from build123d import *

# Parameters (mm, degrees)
SKETCH_R  = 0.48
SKETCH_W  = 22.3
SKETCH_H  = 12.8
PAD_DEPTH = 4.5


with BuildPart() as part:
    # Sketch → Pad (new body)
    with BuildSketch(Plane.XY):
        with BuildLine():
            Line((-17.15, -12.4), (14.15, -12.4))
            ThreePointArc((14.15, -12.4), (16.27132, -11.52132), (17.15, -9.4))
            Line((17.15, -9.4), (17.15, 10.741965))
            ThreePointArc((17.15, 10.741965), (16.27132, 12.863286), (14.15, 13.741965))
            Line((14.15, 13.741965), (-17.15, 13.741965))
            ThreePointArc((-17.15, 13.741965), (-45.41951, 11.467422), (-72.4, 2.727178))
            ThreePointArc((-72.4, 2.727178), (-72.770186, -2.524876), (-68.15, -1e-06))
            ThreePointArc((-17.15, -12.4), (-41.755087, -2.51931), (-68.15, -1e-06))
        make_face()
        with Locations((-13.65, 0)):
            Circle(SKETCH_R, mode=Mode.SUBTRACT)
        with Locations((13.65, 0)):
            Circle(SKETCH_R, mode=Mode.SUBTRACT)
        Rectangle(SKETCH_W, SKETCH_H, mode=Mode.SUBTRACT)
        with BuildLine():
            Line((-17.44, 6.580017), (-17.44, -6.814013))
            ThreePointArc((-19.71, -8.17), (-18.190253, -8.136095), (-17.44, -6.814013))
            ThreePointArc((-19.71, -8.17), (-34.392185, -1.83077), (-49.944735, 1.893553))
            ThreePointArc((-50.141709, 5.809641), (-51.645768, 3.770991), (-49.944735, 1.893553))
            ThreePointArc((-20.45, 9.58), (-35.411915, 8.608801), (-50.141709, 5.809641))
            ThreePointArc((-17.44, 6.580017), (-18.322218, 8.70487), (-20.45, 9.58))
        make_face(mode=Mode.SUBTRACT)
    extrude(amount=PAD_DEPTH)


solid = part.part
Could you check a few things on this model? Use its own coordinates, in mm. A direction names the side the tool comes from. Round coordinates to 2 decimals unless told otherwise and drop trailing zeros. Order: outer loops, then holes, each group sorted by start corner. A loop starts at its lowest first (then second) coordinate and runs counter-clockwise, first axis right, second up.
(1) If we mould it in two halves opening along Y, with no side actions, what happens to faces 1 (the cylindrical face through (-41.39, -2.61, 2.22)), 2 (the flat face through (17.15, 1, 2)), 3 (the cylindrical face through (-51.647, 3.809, 2.218))? For each: released by +Y, released by -Y, zero draft, split by the parting line, or undercut.
Response values:
face 1: released by -Y
face 2: zero draft
face 3: undercut
(2) Imagine slicing it at C-C (x = -32.5). Write out the boundary of the cut face in (y, z), plus the area to 3 significant figures.
Response values:
outline: (-5.29, 0) - (-2.48, 0) - (-2.48, 4.5) - (-5.29, 4.5) - close; (8.94, 0) - (13.33, 0) - (13.33, 4.5) - (8.94, 4.5) - close
area: 32.4 mm2
(3) Imagine slicing it at B-B (x = -5.5). Write out the boundary of the cut face in (y, z).
Response values:
outline: (-12.4, 0) - (-6.4, 0) - (-6.4, 4.5) - (-12.4, 4.5) - close; (6.4, 0) - (13.74, 0) - (13.74, 4.5) - (6.4, 4.5) - close
(4) Imagine slicing it at A-A (z = 1.3). Write out the boundary of the cut face in (x, y), plus the area to 3 significant figures.
Response values:
outline: (-72.4, 2.73) arc R3 ccw (long way) to (-68.15, 0) arc R92.8 cw to (-17.15, -12.4) - (14.15, -12.4) arc R3 ccw to (17.15, -9.4) - (17.15, 10.74) arc R3 ccw to (14.15, 13.74) - (-17.15, 13.74) arc R122 ccw to start; hole (-50.14, 5.81) arc R2 ccw to (-49.94, 1.89) arc R92.8 cw to (-19.71, -8.17) arc R1.54 ccw to (-17.44, -6.81) - (-17.44, 6.58) arc R3 ccw to (-20.45, 9.58) arc R122 ccw to start; hole circle Ø0.96 at (-13.65, 0); hole (-11.15, -6.4) - (11.15, -6.4) - (11.15, 6.4) - (-11.15, 6.4) - close; hole circle Ø0.96 at (13.65, 0)
area: 1,020 mm2
(5) I'm going to push flat-ended pins straight in: pin 1 (1.3 mm diameter, centred on y = 1, z = 1.5, fed in from -X); pin 2 (1.5 mm diameter, centred on x = -2.5, z = 2.5, fed in from +Y); pin 3 (2 mm diameter, centred on x = -64, z = 1.5, fed in from -Y). Where does each tip first touch, or does it pass through?
Response values:
pin 1: stops at x = -74.13
pin 2: stops at y = 13.74
pin 3: stops at y = 0.1
(6) Which directions (+Z, -Z, +X, -X, +Y, -Y) give clear straight access to the entire face, cutting with the end or side of a thin tool? Please do faces 4 (the flat face through (-1, 13.742, 2)), 5 (the flat face through (-2, -12.4, 2)), 6 (the cylindrical face through (-34.18, -1.9, 2.22)).
Response values:
face 4: +Z, -Z, +X, +Y
face 5: +Z, -Z, +X, -X, -Y
face 6: +Z, -Z
(7) Imagine slicing it at D-D (y = 12). Write out the boundary of the cut face in (x, z).
Response values:
outline: (-42.57, 0) - (16.87, 0) - (16.87, 4.5) - (-42.57, 4.5) - close
(8) Please list where these lines run through material, in increasing order: line 1 along Y through (x, z) = (-13.65, 2.8); line 2 along Y through (x, z) = (-6, 1.6); line 3 along Y through (x, z) = (-12, 3.1).
Response values:
line 1: y = -12.4 to -0.48, 0.48 to 13.74
line 2: y = -12.4 to -6.4, 6.4 to 13.74
line 3: y = -12.4 to 13.74
